```python
from build123d import *

# Parameters (mm, degrees)
F2_R = 2.413
F3_R = 3.175


with BuildPart() as f1:
    # F0 (on Front) → F1 (revolve)
    with BuildSketch(Plane.XZ):
        Polygon((-106.3625, 70.612), (-106.3625, 69.85), (-100.0125, 69.85), (-100.0125, 0), (0, 0), (0, 0.762), (-99.2505, 0.762), (-99.2505, 70.612), align=None)
    revolve(axis=Axis((0, 0, 33.215944), (0, 0, 1)))

    # F2
    f2_edges = [f1.edges().sort_by_distance(p)[0] for p in [
        (99.2505, 0, 0.762),
    ]]
    fillet(f2_edges, radius=F2_R)

    # F3
    f3_edges = [f1.edges().sort_by_distance(p)[0] for p in [
        (100.0125, 0, 0),
    ]]
    fillet(f3_edges, radius=F3_R)


solid = f1.part
```
Design review of the part built by this model. Coordinates are the model's own, in mm. A direction names the side the tool comes from. Give positions to 0.01 mm unless a question says otherwise; leave off trailing zeros. Order: outer loops, then holes, each group sorted by start corner. A loop starts at its lowest first (then second) coordinate and runs counter-clockwise, first axis right, second up. Notation, with made-up numbers: M 7.5,29 L 40.5,29 A17 ccw 40.5,36 Z; hole C 60.25,-16 d1. An arc over 180 degrees is marked long. One line per question, with ' | ' between items. Start each with the question number.
Q1. We need section B-B (z = 55.5). Write out the cut boundary in (x, y) (1 decimal), plus the area to 3 significant figures.
Q2. For pin 1 Ø2 at (y, z) = (-7.5, 22) entering from -X; pin 2 Ø3 at (x, y) = (59, -24) entering from +Z; pin 3 Ø5 at (x, z) = (-31, 30) entering from -Y, all flat-tipped, find the tip position at first contact; note any pin that passes through.
Q3. The part is to be moulded in two halves that separate along Y. For faces 4 (the face through (-98.25, 40.74, 70.23)), 5 (the face through (-87.2, -47.8, 70.612)), 6 (the face through (21.52, 96.89, 37.37)), say which applies: +Y half, -Y half, draft (parallel to the pull), parting line (faces both ways), or undercut.
Q4. For L1, parallel to Y at x = 0, z = 56; L2, parallel to Z at x = 70.5, y = -57.5, list the stretches that pass through material, from the lowest coordinate up. Write a range as [from, to].
Q5. Machinability: for faces 1 (the face through (-1, -1, 0.762)), 2 (the face through (21.681, 97.634, 36.046)), 3 (the face through (1, -1, 0)), which of the approach directions +Z, -Z, +X, -X, +Y, -Y give a long, thin tool a straight path to every point of the face, cutting with its end or side? Answer none if there is none.
Returned:
1) outline: C 0,0 d200; hole C 0,0 d198.5 | area: 477 mm2
2) pin 1: x = -99.8 | pin 2: z = 0.76 | pin 3: y = -95.87
3) face 4: parting line | face 5: draft | face 6: undercut
4) L1: [-100.01, -99.25], [99.25, 100.01] | L2: [0, 0.76]
5) face 1: +Z | face 2: -Z | face 3: -Z, +X, -X, +Y, -Y
